Input: part model. Units: mm. Frame: model coordinates. A direction names the side the tool comes from. Coordinates: 2 decimals unless noted, no trailing zeros. Loops run counter-clockwise (first coordinate to the right, second up) from the corner with the lowest first, then second, coordinate; pieces in that order, holes last. Notation, with made-up numbers: M -40,17 L -36,17 A6 cw -36,21 Z; hole C 23,87 d3. An arc over 180 degrees is marked long. Use a Markdown table: item, result. Add a question column.
1. Section A-A on z = 23. Output: boundary loops of the cut face in (x, y), then the cut area to 3 significant figures.
2. Set-up query: faces 4 (the flat face through (1.5, -5, 14.8)), 5 (the cylindrical face through (1.301, 9.285, 14.93)). Return all of +Z, -Z, +X, -X, +Y, -Y with unobstructed straight access to the full face (end or side cutting, diameter ignored); none if empty.
3. Section B-B on y = -2. Output: boundary loops of the cut face in (x, z).
4. Line query: L1, parallel to Y at x = 1.7, z = 23.25; L2, parallel to Y at x = 1.95, z = 4.5; L3, parallel to X at y = 6, z = 4.75. Output: solid intervals per line, ascending. Write a range as [from, to].
5. Draft query along X for faces 1 (the flat face through (1, 3, 15)), 2 (the flat face through (2, 2, 15)), 3 (the cylindrical face through (1.892, 9.512, 25.07)). Return one class per face: +X half, -X half, draft (parallel to the pull), parting line (faces both ways), or undercut.
6. Pin query (flat end, axial travel): pin 1 (4 mm diameter, centred on y = 1.5, z = 21, fed in from +X). Return the tip coordinate at first contact, or that it passes through.
7. Section C-C on y = 1.5. Output: boundary loops of the cut face in (x, z), then the cut area to 3 significant figures.
8. Section D-D on z = 16.75. Output: boundary loops of the cut face in (x, y), then the cut area to 3 significant figures.
Autodesk Inventor part; units mm, degrees
ref_plane "YZ Plane" through (0, 0, 0) normal (1, 0, 0) x (0, 1, 0)
ref_plane "XZ Plane" through (0, 0, 0) normal (0, 1, 0) x (-1, 0, 0)
ref_plane "XY Plane" through (0, 0, 0) normal (0, 0, 1) x (1, 0, 0)
sketch "Szkic1" plane through (0, 0, 0) normal (0, 0, 1) x (1, 0, 0)
  line L0 (2, 10) -> (1, 10)
  line L1 (1, 10) -> (1, -5)
  line L2 (1, -5) -> (2, -5)
  line L3 (2, -5) -> (2, 10)
  circle A0 centre (2, 10) radius 1
  point P0 (0, 0)
  point P1 (0, 0)
  point P2 (2, 9)
  point P3 (2, 9)
extrude "Wyciągnięcie proste1" add sketch "Szkic1" along normal blind 30
ref_plane "Płaszczyzna konstrukcyjna1" through (0, 0, 10) normal (0, 0, 1) x (1, 0, 0)
sketch "Szkic2" plane through (0, 0, 10) normal (0, 0, 1) x (1, 0, 0)
  arc A0 (2, 9) -> (1, 10) centre (2, 10) ccw
  circle A1 centre (2, 10) radius 1
  point P0 (0, 0)
extrude "Wyciągnięcie proste2" cut sketch "Szkic2" along normal blind 10
sketch "Szkic3" plane through (0, 0, 30) normal (0, 0, 1) x (1, 0, 0)
  circle A0 centre (2, 10) radius 0.5
  point P0 (0, 0)
  dimension "d5" = 1
extrude "Wyciągnięcie proste3" cut sketch "Szkic3" against normal blind 30
sketch "Szkic8" plane through (1, -5, 0) normal (-1, 0, 0) x (0, 0, 1)
  point P0 (7, 3)
hole "Otwór5" at (1, -2, 7) direction (1, 0, 0) diameter 2.4 end through all countersink diameter 4.4 countersink angle 90
sketch "Szkic9" plane through (1, -5, 0) normal (-1, 0, 0) x (0, 0, 1)
  point P0 (7, 12)
hole "Otwór6" at (1, 7, 7) direction (1, 0, 0) diameter 2.4 end through all countersink diameter 4.4 countersink angle 90
sketch "Szkic10" plane through (1, -5, 0) normal (-1, 0, 0) x (0, 0, 1)
  point P0 (23, 12)
hole "Otwór7" at (1, 7, 23) direction (1, 0, 0) diameter 2.4 end through all countersink diameter 4.4 countersink angle 90
sketch "Szkic11" plane through (1, -5, 0) normal (-1, 0, 0) x (0, 0, 1)
  point P0 (23, 3)
hole "Otwór8" at (1, -2, 23) direction (1, 0, 0) diameter 2.4 end through all countersink diameter 4.4 countersink angle 90
properties part number "hinge 2"
Answers below:
| question | item | result |
|---|---|---|
| 1 | outline | M 1,-5 L 2,-5 L 2,-3.2 L 1,-4.2 Z; M 1,0.2 L 2,-0.8 L 2,5.8 L 1,4.8 Z; M 1,9.2 L 2,8.2 L 2,9 A1 ccw long 1,10 Z; hole C 2,10 d1 |
| 1 | area | 9.77 mm² |
| 2 | face 4 | +Z, -Z, +X, -X, -Y |
| 2 | face 5 | +X, +Y |
| 3 | outline | M 1,0 L 2,0 L 2,5.8 L 1,4.8 Z; M 1,9.2 L 2,8.2 L 2,21.8 L 1,20.8 Z; M 1,25.2 L 2,24.2 L 2,30 L 1,30 Z |
| 4 | L1 | y = [-5, -3.48], [-0.52, 5.52], [8.48, 9.6], [10.4, 10.95] |
| 4 | L2 | y = [-5, 9.5], [10.5, 11] |
| 4 | L3 | x = [1, 2] |
| 5 | face 1 | -X half |
| 5 | face 2 | +X half |
| 5 | face 3 | undercut |
| 6 | pin 1 | stops at x = 2 |
| 7 | outline | M 1,0 L 2,0 L 2,30 L 1,30 Z |
| 7 | area | 30.0 mm² |
| 8 | outline | M 1,-5 L 2,-5 L 2,9 A1 cw 1,10 Z |
| 8 | area | 14.2 mm² |
